```python
from build123d import *

# Parameters (mm, degrees)
BOSS_EXTRU_1_DEPTH = 10
CONG_1_R           = 10


with BuildPart() as part:
    # Esquisse1 → Boss.-Extru.1 (new body)
    with BuildSketch(Plane.XY):
        with BuildLine():
            ThreePointArc((75, 0), (0, -75), (-75, 0))
            Line((-75, 0), (-75, -162.276597369))
            ThreePointArc((-75, -162.276597369), (0, -87.276597369), (75, -162.276597369))
            Line((75, -162.276597369), (75, 0))
        make_face()
        with BuildLine():
            ThreePointArc((75, 0), (0, 75), (-75, 0))
            Line((-75, 0), (75, 0))
        make_face()
        with BuildLine():
            Line((75, 0), (-75, 0))
            ThreePointArc((-75, 0), (0, -75), (75, 0))
        make_face()
        with BuildLine():
            ThreePointArc((75, -162.276597369), (0, -87.276597369), (-75, -162.276597369))
            Line((-75, -162.276597369), (75, -162.276597369))
        make_face()
        with BuildLine():
            Line((75, -162.276597369), (-75, -162.276597369))
            ThreePointArc((-75, -162.276597369), (0, -237.276597369), (75, -162.276597369))
        make_face()
    extrude(amount=BOSS_EXTRU_1_DEPTH)

    # Congé1
    cong_1_edges = [part.edges().sort_by_distance(p)[0] for p in [
        (0, 75, 10),
        (75, -81.138298684, 10),
        (0, -237.276597369, 10),
        (-75, -81.138298684, 10),
    ]]
    fillet(cong_1_edges, radius=CONG_1_R - 0.0001)  # a hair under: the kernel refuses the full size


solid = part.part
```
Could you check a few things on this model? Use its own coordinates, in mm. Coordinates: 2 decimals unless noted, no trailing zeros. Write each loop counter-clockwise with the first axis right and the second up, starting at its lowest first coordinate (ties: lowest second). Pieces come first, ordered by that corner, then holes. Notation, with made-up numbers: (-29, 38.25) -> (-24, 38.25) arc R11 cw to (-24, 45.25) -> close; hole circle Ø9 at (65, -8.5). An arc over 180 degrees is marked (long way). One line per question, with ' | ' between items. Start each with the question number.
1. Will these pins go through, and if not, where does the flat tip stop? P1, Ø5, axis at x = -27.5, z = 3.5, coming from the -Y side; P2, Ø5, axis at x = 57, z = 2, coming from the -Y side; P3, Ø1.5, axis at y = -33.5, z = 3, coming from the -X side.
2. Please list where these lines run through material, in increasing order: line 1 along Y through (x, z) = (-24, 9); line 2 along X through (y, z) = (-158.5, 5); line 3 along X through (y, z) = (-29, 2).
3. If we section it at B-B (z = 2.5): Please give me the cut outline in (x, y).
Return value:
1) P1: stops at y = -232.6 | P2: stops at y = -213.58 | P3: stops at x = -74.74
2) line 1: y = -227.35 to 65.07 | line 2: x = -73.66 to 73.66 | line 3: x = -74.8 to 74.8
3) outline: (-74.68, -162.28) arc R74.68 ccw to (74.68, -162.28) -> (74.68, 0) arc R74.68 ccw to (-74.68, 0) -> close
